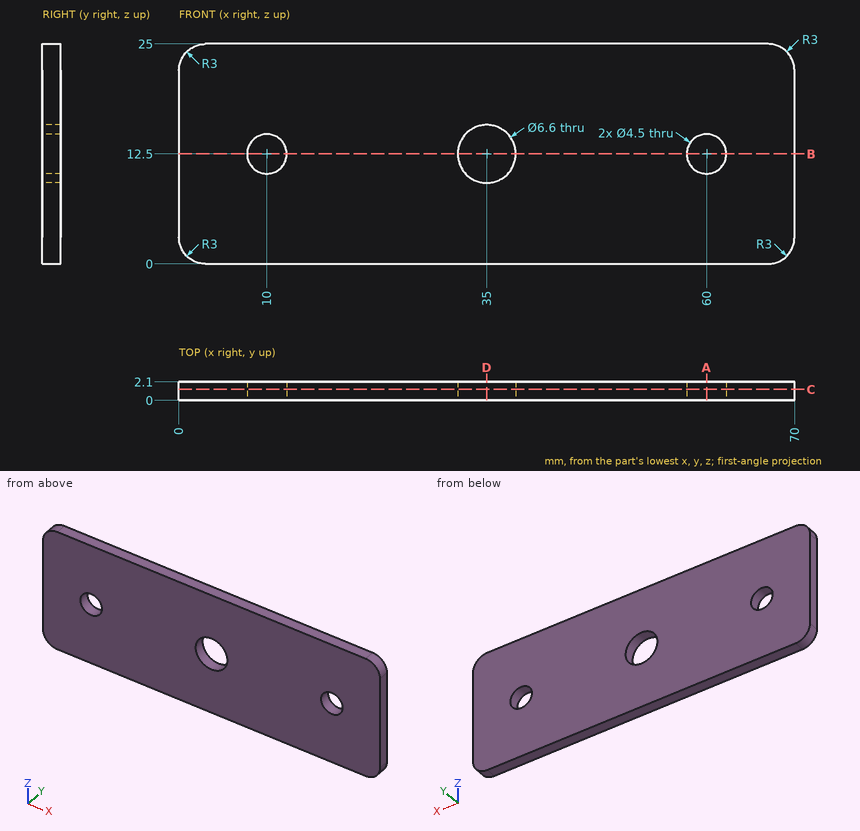
The figure shows three views and two pictorial views of one solid part (mm, origin at its lowest corner). Answer the questions. Coordinates: 2 decimals unless noted, no trailing zeros. Order: outer loops, then holes, each group sorted by start corner. A loop starts at its lowest first (then second) coordinate and runs counter-clockwise, first axis right, second up.
Q1. Given P1, Ø10, axis at x = 63, z = 3.5, coming from the -Y side; P2, Ø3.5, axis at x = 60, z = 12.5, coming from the -Y side, each flat-ended and moving along its own axis, determine where each tip first touches the part or whether it passes through.
Q2. A cutting plane is placed at A-A, the plane x = 60. Write down the section's boundary in (y, z), and give its area (4 significant figures).
Q3. A cutting plane is placed at B-B, the plane z = 12.5. Write down the section's boundary in (x, y).
Q4. A cutting plane is placed at D-D, the plane x = 35. Write down the section's boundary in (y, z).
Q5. Consider line 1 (X direction, y = 0.8, z = 12.5); line 2 (Z direction, x = 10, y = 1.35); line 3 (Z direction, x = 35, y = 0.75). Determine where each line is inside the solid, lowest interval first.
Q6. A cutting plane is placed at C-C, the plane y = 1.25. Write down the section's boundary in (x, z), and give its area (3 significant figures).
Answers follow:
1. P1: stops at y = 0
1. P2: passes through
2. outline: (0, 0) - (2.1, 0) - (2.1, 10.25) - (0, 10.25) - close; (0, 14.75) - (2.1, 14.75) - (2.1, 25) - (0, 25) - close
2. area: 43.05 mm2
3. outline: (0, 0) - (7.75, 0) - (7.75, 2.1) - (0, 2.1) - close; (12.25, 0) - (31.7, 0) - (31.7, 2.1) - (12.25, 2.1) - close; (38.3, 0) - (57.75, 0) - (57.75, 2.1) - (38.3, 2.1) - close; (62.25, 0) - (70, 0) - (70, 2.1) - (62.25, 2.1) - close
4. outline: (0, 0) - (2.1, 0) - (2.1, 9.2) - (0, 9.2) - close; (0, 15.8) - (2.1, 15.8) - (2.1, 25) - (0, 25) - close
5. line 1: x = 0 to 7.75, 12.25 to 31.7, 38.3 to 57.75, 62.25 to 70
5. line 2: z = 0 to 10.25, 14.75 to 25
5. line 3: z = 0 to 9.2, 15.8 to 25
6. outline: (0, 3) arc R3 ccw to (3, 0) - (67, 0) arc R3 ccw to (70, 3) - (70, 22) arc R3 ccw to (67, 25) - (3, 25) arc R3 ccw to (0, 22) - close; hole circle Ø4.5 at (10, 12.5); hole circle Ø6.6 at (35, 12.5); hole circle Ø4.5 at (60, 12.5)
6. area: 1,680 mm2
